Design review of the part built by this model. Coordinates are the model's own, in mm. Face numbers are marked on the shaded views. A direction names the side the tool comes from. Round coordinates to 2 decimals unless told otherwise and drop trailing zeros. Loops run counter-clockwise (first coordinate to the right, second up) from the corner with the lowest first, then second, coordinate; pieces in that order, holes last. Notation, with made-up numbers: (50, -3.75) - (107, -3.75) arc R14 ccw to (107, 15.25) - close; hole circle Ø3 at (51.5, 2.5). An arc over 180 degrees is marked (long way). Return JSON: item names as keys, results as strings. Group by question number.
Autodesk Inventor part; units mm, degrees
ref_plane "YZ Plane" through (0, 0, 0) normal (1, 0, 0) x (0, 1, 0)
ref_plane "XZ Plane" through (0, 0, 0) normal (0, 1, 0) x (-1, 0, 0)
ref_plane "XY Plane" through (0, 0, 0) normal (0, 0, 1) x (1, 0, 0)
sketch "Sketch1" plane through (0, 0, 0) normal (0, 0, 1) x (1, 0, 0)
  line L0 (0, 0) -> (25, 0)
  line L1 (25, 0) -> (25, 40)
  line L2 (25, 40) -> (0, 40)
  line L3 (0, 40) -> (0, 0)
  dimension "d1" = 25
  dimension "d2" = 40
  dimension "d3" = 25
extrude "Extrusion1" add sketch "Sketch1" against normal blind 30
sketch "Sketch2" plane through (25, 0, 0) normal (1, 0, 0) x (0, 0, -1)
  line L0 (0, 0) -> (30, 0)
  circle A0 centre (15, 6.56) radius 2.46
extrude "Extrusion2" cut sketch "Sketch2" against normal blind 30
sketch "Sketch3" plane through (0, 0, 0) normal (-1, 0, 0) x (0, 0, 1)
  line L0 (0, 0) -> (-30, 0)
  line L1 (-25.05, 0) -> (-4.95, 0)
  line L2 (-4.95, 0) -> (-4.95, 33.12)
  line L3 (-4.95, 33.12) -> (-25.05, 33.12)
  line L4 (-25.05, 33.12) -> (-25.05, 0)
  dimension "d11" = 20.1
extrude "Extrusion3" cut sketch "Sketch3" against normal blind 20
sketch "Sketch4" plane through (0, 0, 0) normal (0, -1, 0) x (1, 0, 0)
  line L0 (20, -4.95) -> (20, -25.05)
  line L1 (20, -15) -> (25, -15)
  line L2 (25, 0) -> (25, -30)
  line L3 (20, -8.025) -> (25, -8.025)
  line L4 (25, -8.025) -> (25, -21.975)
  line L5 (25, -21.975) -> (20, -21.975)
  line L6 (20, -21.975) -> (20, -8.025)
  line L7 (20, -8.025) -> (25, -21.975) construction
  line L8 (25, -8.025) -> (20, -21.975) construction
  line L9 (25, -12.54) -> (25, -17.46)
  point P0 (0, 0)
  point P1 (22.5, -15)
  dimension "d14" = 13.95
extrude "Extrusion4" add sketch "Sketch4" along normal blind 15
sketch "Sketch5" plane through (20, 0, 0) normal (-1, 0, 0) x (0, 0, 1)
  circle A0 centre (-15, 6.56) radius 2.46
  circle A1 centre (-15, 6.56) radius 4.7025
  circle A2 centre (-15, 6.56) radius 2.46
  circle A3 centre (-15, 6.56) radius 2.46
  point P0 (0, 0)
  dimension "d17" = 9.405
extrude "Extrusion5" cut sketch "Sketch5" against normal blind 2.1
sketch "Sketch6" plane through (25, 0, 0) normal (1, 0, 0) x (0, 0, -1)
  circle A0 centre (15, 6.56) radius 4.7025
  line L0 (15, 6.56) -> (15, 23.56)
  circle A1 centre (15, 23.56) radius 2.46
  point P0 (0, 0)
  dimension "d20" = 17
  dimension "d21" = 4.92
extrude "Extrusion6" cut sketch "Sketch6" against normal blind 10 contours A1
sketch "Sketch7" plane through (20, 0, 0) normal (-1, 0, 0) x (0, 0, 1)
  circle A0 centre (-15, 23.56) radius 2.46
  circle A1 centre (-15, 23.56) radius 4.7025
  point P0 (0, 0)
  dimension "d24" = 9.405
extrude "Extrusion7" cut sketch "Sketch7" against normal blind 2.1
sketch "Sketch9" plane through (25, 0, 0) normal (1, 0, 0) x (0, 0, -1)
  circle A0 centre (15, 6.56) radius 2.46
  circle A1 centre (15, 6.56) radius 2.46
  circle A2 centre (15, 23.56) radius 2.46
  circle A3 centre (15, 23.56) radius 2.46
  line L0 (30, 40) -> (30, 0)
  line L1 (30, 0) -> (30, 40)
  line L2 (30, 40) -> (0, 40)
  line L3 (0, 40) -> (0, 0)
  line L4 (0, 0) -> (8.025, 0)
  line L5 (21.975, 0) -> (21.975, -15)
  line L6 (21.975, -15) -> (8.025, -15)
  line L7 (8.025, -15) -> (8.025, 0)
  line L8 (0, 0) -> (8.025, 0)
  line L9 (21.975, 0) -> (30, 0)
extrude "Extrusion8" add sketch "Sketch9" along normal blind 5
sketch "Sketch10" plane through (0, 40, 0) normal (0, 1, 0) x (1, 0, 0)
  line L0 (0, 30) -> (30, 30)
  line L1 (30, 0) -> (0, 0)
  line L2 (0, 30) -> (30, 30)
  line L3 (30, 30) -> (30, 0)
  line L4 (30, 0) -> (0, 0)
  line L5 (0, 0) -> (0, 30)
extrude "Extrusion9" add sketch "Sketch10" along normal blind 30
sketch "Sketch12" plane through (30, 0, 0) normal (1, 0, 0) x (0, 0, -1)
  circle A0 centre (15, 6.56) radius 2.46
  line L0 (15, 6.56) -> (15, 15.06)
  circle A1 centre (15, 15.06) radius 2.525
  point P0 (0, 0)
  dimension "d31" = 8.5
  dimension "d33" = 5.05
extrude "Extrusion10" cut sketch "Sketch12" against normal blind 30 contours A1
sketch "Sketch14" plane through (0, 0, 0) normal (0, 0, 1) x (1, 0, 0)
  line L0 (30, 70) -> (0, 70)
  line L1 (0, 70) -> (0, 85)
  line L2 (30, 0) -> (30, 70)
  line L3 (30, 113) -> (30, 70)
  line L4 (30, 105) -> (30, 100)
  line L5 (-12, 128) -> (15, 128)
  line L6 (-8, 126) -> (-12, 128)
  line L7 (-8, 126) -> (-4, 114)
  line L8 (-8, 102) -> (-12, 100)
  line L9 (-8, 102) -> (-4, 114)
  line L10 (30, 113) -> (15, 128)
  line L11 (0, 100) -> (-12, 100)
  line L12 (0, 100) -> (0, 85)
  point P0 (0, 0)
  dimension "d69" = 28
  dimension "d74" = 12
extrude "Extrusion12" add sketch "Sketch14" against normal blind 30
sketch "Sketch15" plane through (0, 0, -25.05) normal (-1, 0, 0) x (0, 0, 1)
  line L0 (0, 33.12) -> (20.1, 33.12)
  line L1 (20.1, 33.12) -> (20.1, 0)
  line L2 (0, 33.12) -> (20.1, 33.12)
  line L3 (20.1, 33.12) -> (20.1, 31.1)
  line L4 (20.1, 31.1) -> (0, 31.1)
  line L5 (0, 31.1) -> (0, 33.12)
  point P0 (25.05, 0)
  dimension "d57" = 2.02
extrude "Extrusion13" add sketch "Sketch15" against normal blind 20
properties part number "24mm_x_30mm"
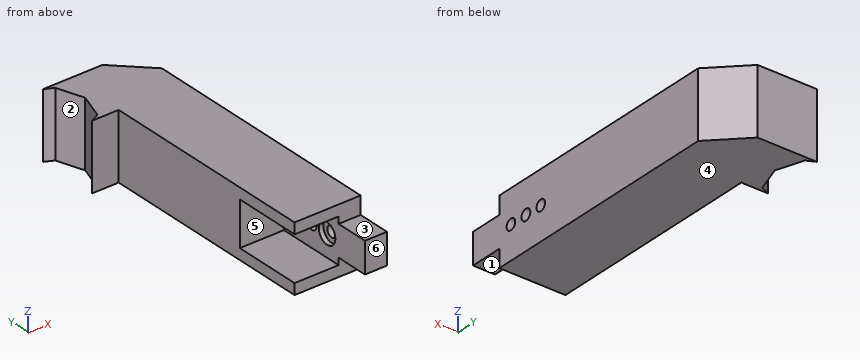
Q1. For line 1 (Y direction, x = 21.5, z = -15) (1 decimal); line 2 (Y direction, x = 21.1, z = -15) (1 decimal); line 3 (Z direction, x = 22, y = 15.06) (3 decimals), list the stretches that pass through material, from the lowest coordinate up.
Q2. Add section C-C, the plane x = 17. State the section outline as (y, z) points.
Q3. Draft analysis for pull direction Z (two halves, no side actions). For the marked faces 4, 5 and 6, state which applies: pulls with the +Z half, pulls with the -Z half, needs draft (parallel to the pull), parting line crosses it, or undercut.
Q4. Add section B-B, the plane z = -15. Give the number of separate pieces and of enclosed holes in the cut face, plus the area to 3 significant figures.
Q5. Add section A-A, the plane y = 23.56. State the section outline as (x, z) points, plus the area to 3 significant figures.
Q6. Add section D-D, the plane y = -5. State the section outline as (x, z) points (3 decimals).
Q7. Insertion check: pin 1 Ø8.5 at (y, z) = (23.56, -15) entering from -X; pin 2 Ø16 at (y, z) = (2, -14.5) entering from -X; pin 3 Ø9 at (y, z) = (66.5, -18.5) entering from -X; pin 4 Ø4 at (y, z) = (23.56, -15) entering from +X. Each pin has a flat end and moves straight along its axis. Give the tip position at first contact, or say it passes through.
Q8. Tool access review of the marked faces 1, 2 and 3: name each direction out of +Z, -Z, +X, -X, +Y, -Y from which nothing blocks a thin tool from reaching the whole face with its end or side.
Evaluation:
{
 "1": {"line 1": "-15 to 1.9, 11.3 to 12.5, 17.6 to 18.9, 28.3 to 121.5", "line 2": "-15 to 1.9, 11.3 to 12.5, 17.6 to 18.9, 28.3 to 121.9", "line 3": "-30 to -17.525, -12.475 to 0"},
 "2": {"outline": "(0, -30) - (126, -30) - (126, 0) - (0, 0) - (0, -4.95) - (31.1, -4.95) - (31.1, -25.05) - (0, -25.05) - close"},
 "3": {"face 4": "pulls with the -Z half", "face 5": "undercut", "face 6": "needs draft"},
 "4": {"separate pieces": "4", "enclosed holes": "0", "area": "3,270 mm²"},
 "5": {"outline": "(0, -30) - (30, -30) - (30, -17.46) - (22.1, -17.46) - (22.1, -19.7) - (20, -19.7) - (20, -25.05) - (0, -25.05) - close; (0, -4.95) - (20, -4.95) - (20, -10.3) - (22.1, -10.3) - (22.1, -12.54) - (30, -12.54) - (30, 0) - (0, 0) - close", "area": "439 mm²"},
 "6": {"outline": "(20, -21.975) - (30, -21.975) - (30, -8.025) - (20, -8.025) - close"},
 "7": {"pin 1": "x = 22.1", "pin 2": "x = 20", "pin 3": "x = 0", "pin 4": "through"},
 "8": {"face 1": "-Z, +X, -X, -Y", "face 2": "+Z, -Z, -X", "face 3": "+Z, +X, -X, -Y"}
}
